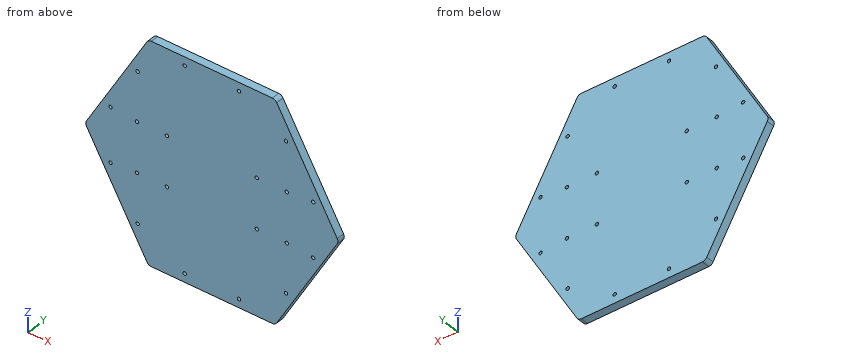
from build123d import *

# Parameters (mm, degrees)
SKETCH1_R          = 1.7
BASE_FLANGE1_DEPTH = 8
FILLET2_R          = 5


# Sheet-metal steps are written as plain solids
with BuildPart() as part:
    # Sketch1 → Base-Flange1 (new body)
    with BuildSketch(Plane(origin=(0, 0, 0), x_dir=(1, 0, 0), z_dir=(0, 1, 0))):
        Polygon((127.017059222, 0), (63.508529611, 110), (-63.508529611, 110), (-127.017059222, 0), (-63.508529611, -110), (63.508529611, -110), align=None)
        with Locations(Location((-75, 25, 0), (0, 0, 270))):
            Circle(SKETCH1_R, mode=Mode.SUBTRACT)
        with Locations(Location((-75, -25, 0), (0, 0, 270))):
            Circle(SKETCH1_R, mode=Mode.SUBTRACT)
        with Locations(Location((75, 25, 0), (0, 0, 270))):
            Circle(SKETCH1_R, mode=Mode.SUBTRACT)
        with Locations(Location((75, -25, 0), (0, 0, 270))):
            Circle(SKETCH1_R, mode=Mode.SUBTRACT)
        with Locations(Location((-45, 25, 0), (0, 0, 270))):
            Circle(SKETCH1_R, mode=Mode.SUBTRACT)
        with Locations(Location((-45, -25, 0), (0, 0, 270))):
            Circle(SKETCH1_R, mode=Mode.SUBTRACT)
        with Locations(Location((45, 25, 0), (0, 0, 270))):
            Circle(SKETCH1_R, mode=Mode.SUBTRACT)
        with Locations(Location((45, -25, 0), (0, 0, 270))):
            Circle(SKETCH1_R, mode=Mode.SUBTRACT)
        with Locations(Location((-74.246212025, -74.246212025, 0), (0, 0, 270))):
            Circle(SKETCH1_R, mode=Mode.SUBTRACT)
        with Locations(Location((-101.42221176, -27.175999736, 0), (0, 0, 270))):
            Circle(SKETCH1_R, mode=Mode.SUBTRACT)
        with Locations(Location((-101.42221176, 27.175999736, 0), (0, 0, 270))):
            Circle(SKETCH1_R, mode=Mode.SUBTRACT)
        with Locations(Location((-74.246212025, 74.246212025, 0), (0, 0, 270))):
            Circle(SKETCH1_R, mode=Mode.SUBTRACT)
        with Locations(Location((-27.175999736, 101.42221176, 0), (0, 0, 270))):
            Circle(SKETCH1_R, mode=Mode.SUBTRACT)
        with Locations(Location((27.175999736, 101.42221176, 0), (0, 0, 270))):
            Circle(SKETCH1_R, mode=Mode.SUBTRACT)
        with Locations(Location((74.246212025, 74.246212025, 0), (0, 0, 270))):
            Circle(SKETCH1_R, mode=Mode.SUBTRACT)
        with Locations(Location((101.42221176, 27.175999736, 0), (0, 0, 270))):
            Circle(SKETCH1_R, mode=Mode.SUBTRACT)
        with Locations(Location((101.42221176, -27.175999736, 0), (0, 0, 270))):
            Circle(SKETCH1_R, mode=Mode.SUBTRACT)
        with Locations(Location((74.246212025, -74.246212025, 0), (0, 0, 270))):
            Circle(SKETCH1_R, mode=Mode.SUBTRACT)
        with Locations(Location((27.175999736, -101.42221176, 0), (0, 0, 270))):
            Circle(SKETCH1_R, mode=Mode.SUBTRACT)
        with Locations(Location((-27.175999736, -101.42221176, 0), (0, 0, 270))):
            Circle(SKETCH1_R, mode=Mode.SUBTRACT)
    extrude(amount=-BASE_FLANGE1_DEPTH)

    # Fillet2
    fillet2_edges = [part.edges().sort_by_distance(p)[0] for p in [
        (63.508529611, -4, 110),
        (-63.508529611, -4, 110),
        (-127.017059222, -4, 0),
        (-63.508529611, -4, -110),
        (63.508529611, -4, -110),
        (127.017059222, -4, 0),
    ]]
    fillet(fillet2_edges, radius=FILLET2_R)


solid = part.part
Source: CAD feature listing. Evaluate the final solid. Frame: model axes, mm. Round coordinates to 2 decimals unless told otherwise and drop trailing zeros. Loops run counter-clockwise (first coordinate to the right, second up) from the corner with the lowest first, then second, coordinate; pieces in that order, holes last.
Q1. Section B-B, the plane z = 69.5. Return loops of the section in (x, y).
Q2. Section C-C, the plane z = 12. Return loops of the section in (x, y), plus the area to 3 significant figures.
Q3. First-contact query: P1, Ø2.5, axis at x = 27.18, z = -101.42, coming from the +Y side; P2, Ø1.5, axis at y = -6, z = 60.5, coming from the -X side; P3, Ø3, axis at x = -64, y = -4, coming from the -Z side; P4, Ø3, axis at y = -3.5, z = -30, coming from the -X side. Flat tips, straight axial feed; report the tip coordinate or a pass-through.
Q4. Section A-A, the plane y = -6.75. State how many separate pieces and enclosed holes the cut face has, plus the area to 3 significant figures.
Q5. Ray query, line 1 (Z direction, x = 75, y = -6); line 2 (X direction, y = -2.25, z = -25); line 3 (X direction, y = -6, z = 27). Return the intervals inside material, ascending.
Solutions:
1. outline: (-86.89, -8) - (86.89, -8) - (86.89, 0) - (-86.89, 0) - close
2. outline: (-120.09, -8) - (120.09, -8) - (120.09, 0) - (-120.09, 0) - close
2. area: 1,920 mm2
3. P1: passes through
3. P2: stops at x = -92.52
3. P3: stops at z = -109.63
3. P4: stops at x = -110.56
4. separate pieces: 1
4. enclosed holes: 20
4. area: 41,700 mm2
5. line 1: z = -90.1 to -75.77, -72.72 to -26.7, -23.3 to 23.3, 26.7 to 72.72, 75.77 to 90.1
5. line 2: x = -112.58 to -76.7, -73.3 to -46.7, -43.3 to 43.3, 46.7 to 73.3, 76.7 to 112.58
5. line 3: x = -111.43 to -103.11, -99.73 to 99.73, 103.11 to 111.43
